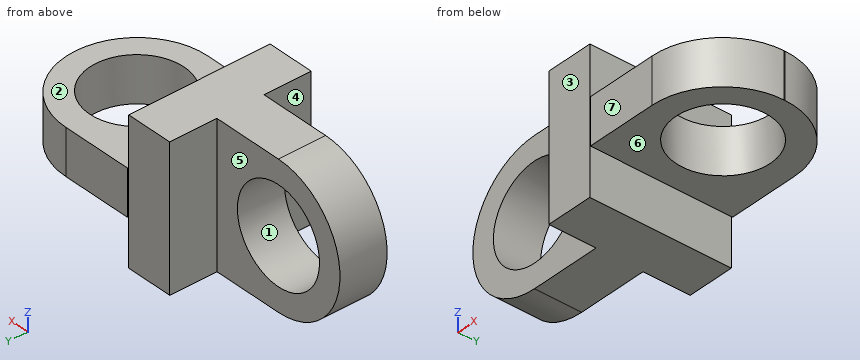
```python
from build123d import *

# Parameters (mm, degrees)
F8_R          = 20
F0_DEPTH      = 10
F0_DEPTH_BACK = 10
F1_W          = 20
F1_H          = 60
F2_DEPTH      = 20
F9_DEPTH      = 60
F6_R          = 20
F10_DEPTH     = 25
F7_R          = 30


with BuildPart() as f0:
    # F8 (on Front) → F0 (new body, two sides)
    with BuildSketch(Plane.XZ) as f0_sk:
        with BuildLine():
            Line((30, 30), (0, 30))
            ThreePointArc((0, 30), (-30, 0), (0, -30))
            Line((0, -30), (30, -30))
            Line((30, -30), (30, 30))
        make_face()
        Circle(F8_R, mode=Mode.SUBTRACT)
    extrude(amount=F0_DEPTH)
    extrude(f0_sk.sketch, amount=-F0_DEPTH_BACK)

    # F1 (on face) → F2 (join)
    with BuildSketch(Plane.YZ.offset(30)):
        with Locations((-20, 0)):
            Rectangle(F1_W, F1_H)
        with Locations((20, 0)):
            Rectangle(F1_W, F1_H)
        Polygon((10, 30), (0, 30), (-10, 30), (-10, -30), (0, -30), (10, -30), align=None)
    extrude(amount=F2_DEPTH)

    # F5 (on offset) → F9 (join)
    with BuildSketch(Plane.YZ.offset(50)):
        Polygon((-29.7670396838, 9.4578760595), (-29.7670396838, -0.5421239405), (-29.7670396838, -9.8316618399), (30.5491250266, -9.8316618399), (30.5491250266, 9.4578760595), align=None)
    extrude(amount=F9_DEPTH)

    # F6 (on face) → F10 (cut)
    with BuildSketch(Plane.XY.offset(9.4578760595)):
        with Locations((80.4655393111, 0)):
            Circle(F6_R)
    extrude(amount=-F10_DEPTH, mode=Mode.SUBTRACT)

    # F7
    f7_edges = [f0.edges().sort_by_distance(p)[0] for p in [
        (110, -29.76704, -0.186893),
        (110, 30.549125, -0.186893),
    ]]
    fillet(f7_edges, radius=F7_R)


solid = f0.part
```
For this review, take the finished solid that the model builds, in its own axes (mm). Face numbers are marked on the shaded views. A direction names the side the tool comes from. Give positions to 0.01 mm unless a question says otherwise; leave off trailing zeros. Write each loop counter-clockwise with the first axis right and the second up, starting at its lowest first coordinate (ties: lowest second). Pieces come first, ordered by that corner, then holes. Notation, with made-up numbers: M -39,59.25 L -33,59.25 A10 ccw -33,67.25 Z; hole C 63.5,29.25 d11. An arc over 180 degrees is marked long. One line per item, written item: value.
1) For line 1 (Z direction, x = 0, y = 0.5); line 2 (X direction, y = -16, z = -22); line 3 (Y direction, x = 13, z = -16), list the stretches that pass through material, from the lowest coordinate up. Write a range as from..to.
Results are:
line 1: z = -30..-20, 20..30
line 2: x = 30..50
line 3: y = -10..10
2) Take a section at C-C, the plane z = 18.5. Write out the cut boundary in (x, y).
Results are:
outline: M -23.62,-10 L -7.6,-10 L -7.6,10 L -23.62,10 Z; M 7.6,-10 L 30,-10 L 30,-30 L 50,-30 L 50,30 L 30,30 L 30,10 L 7.6,10 Z
3) Take a section at D-D, the plane z = -6.5. Write out the cut boundary in (x, y).
Results are:
outline: M -29.29,-10 L -18.91,-10 L -18.91,10 L -29.29,10 Z; M 18.91,-10 L 30,-10 L 30,-30 L 50,-30 L 50,-29.77 L 80,-29.77 A30 ccw 110,0.23 L 110,0.55 A30 ccw 80,30.55 L 50,30.55 L 50,30 L 30,30 L 30,10 L 18.91,10 Z; hole C 80.47,0 d40
4) For P1, Ø6, axis at x = 30.5, z = 0, coming from the +Y side; P2, Ø6, axis at y = 20.5, z = 0.5, coming from the -X side; P3, Ø12, axis at x = -12.5, z = 13.5, coming from the +Y side, all flat-tipped, find the tip position at first contact; note any pin that passes through.
Results are:
P1: stops at y = 30
P2: stops at x = 30
P3: stops at y = 10
5) Take a section at A-A, the plane z = 0. Write out the cut boundary in (x, y), then the cut area to 3 significant figures.
Results are:
outline: M -30,-10 L -20,-10 L -20,10 L -30,10 Z; M 20,-10 L 30,-10 L 30,-30 L 50,-30 L 50,-29.77 L 80,-29.77 A30 ccw 110,0.23 L 110,0.55 A30 ccw 80,30.55 L 50,30.55 L 50,30 L 30,30 L 30,10 L 20,10 Z; hole C 80.47,0 d40
area: 3,580 mm²
6) Take a section at B-B, the plane y = -14. Write out the cut boundary in (x, z), then the cut area to 3 significant figures.
Results are:
outline: M 30,-30 L 50,-30 L 50,-9.83 L 66.18,-9.83 L 66.18,9.46 L 50,9.46 L 50,30 L 30,30 Z; M 94.75,-9.83 L 106.41,-9.83 L 106.41,9.46 L 94.75,9.46 Z
area: 1,740 mm²
7) For the marked faces 4, 5, 6 and 7, list the 3-axis set-ups (+Z, -Z, +X, -X, +Y, -Y) from which the entire face can be reached by the end or side of a thin tool; tool diameter is ignored.
Results are:
face 4: +Z, -Z, -X, -Y
face 5: +Z, -Z, -X, +Y
face 6: -Z, +X, +Y, -Y
face 7: +Z, -Z, +X, -Y
8) The part is to be moulded in two halves that separate along Z. For the marked faces 1, 2 and 3, say which applies: +Z half, -Z half, draft (parallel to the pull), parting line (faces both ways), or undercut.
Results are:
face 1: undercut
face 2: +Z half
face 3: draft
